Input: part model. Units: mm. Frame: model coordinates. Face numbers are marked on the shaded views. Round coordinates to 2 decimals unless told otherwise and drop trailing zeros. Order: outer loops, then holes, each group sorted by start corner. A loop starts at its lowest first (then second) coordinate and runs counter-clockwise, first axis right, second up. Notation, with made-up numbers: (-34.75, 56.5) -> (8.25, 56.5) arc R22 ccw to (8.25, 92.5) -> close; hole circle Ø2 at (-21.75, 58.25). An arc over 180 degrees is marked (long way). Use a Markdown table: item, result.
from build123d import *

# Parameters (mm, degrees)
SKETCH1_W                = 21.59
SKETCH1_H                = 13.97
DEPTH_A_DEPTH            = 6.35
ROUND_EXTRUDE_DEPTH      = 21.59
ANGLE_CUT_DEPTH          = 29.967416609
STRING_HOLE_R            = 0.762
STRING_HOLE_CUT_DEPTH    = 29.967416609
ELASTIC_HOLES_R          = 2.54
ELASTIC_HOLE_CUT_DEPTH   = 29.967416609
FILLET1_R                = 6.35
GUIDE_OUTIE_REACH        = 30.967
SKETCH7_R                = 2.54
ELASTIC_HOLE_CUT_2_DEPTH = 29.967416778


with BuildPart() as part:
    # Sketch1 → depth a (new body)
    with BuildSketch(Plane(origin=(0, 0, 0), x_dir=(1, 0, 0), z_dir=(0, 1, 0))):
        with Locations((-10.795, 6.985)):
            Rectangle(SKETCH1_W, SKETCH1_H)
    extrude(amount=DEPTH_A_DEPTH)

    # Sketch4 → round extrude (add)
    with BuildSketch(Plane(origin=(0, 0, 0), x_dir=(0, 0, -1), z_dir=(1, 0, 0))):
        with BuildLine():
            Line((0, 6.35), (13.97, 6.35))
            ThreePointArc((13.97, 6.35), (6.985, 13.335), (0, 6.35))
        make_face()
    extrude(amount=-ROUND_EXTRUDE_DEPTH)

    # Sketch5 → angle cut (cut, through all)
    with BuildSketch(Plane.XY):
        Polygon((0, 6.35), (0, 13.335), (-6.985, 13.335), align=None)
    extrude(amount=-ANGLE_CUT_DEPTH, mode=Mode.SUBTRACT)

    # string hole → string hole cut (cut, through all)
    with BuildSketch(Plane(origin=(0, 0, 0), x_dir=(0, 0, -1), z_dir=(1, 0, 0))):
        with Locations((6.985, 11.684)):
            Circle(STRING_HOLE_R)
    extrude(amount=-STRING_HOLE_CUT_DEPTH, mode=Mode.SUBTRACT)

    # elastic holes → elastic hole cut (cut, through all)
    with BuildSketch(Plane(origin=(0, 0, 0), x_dir=(0, 0, -1), z_dir=(1, 0, 0))):
        with Locations((3.4925, 3.175)):
            Circle(ELASTIC_HOLES_R)
        with Locations(Location((10.4775, 3.175, 0), (0, 0, 180))):
            Circle(ELASTIC_HOLES_R)
    extrude(amount=-ELASTIC_HOLE_CUT_DEPTH, mode=Mode.SUBTRACT)

    # Fillet1
    # the kernel refuses this fillet: 6.35 mm, written as the material it takes off along each edge
    with BuildSketch(Plane(origin=(-21.59, 6.35, -6.985), x_dir=(0, 0, -1), z_dir=(0, -1, 0))) as fillet1_piece_1:
        with BuildLine():
            CenterArc((6.985 - FILLET1_R, FILLET1_R), FILLET1_R, 270, 90)
            Line((6.985, FILLET1_R), (6.985, 0))
            Line((6.985, 0), (6.985 - FILLET1_R, 0))
        make_face()
    revolve(axis=Axis((-21.59, 6.35, -6.985), (1, 0, 0)), revolution_arc=180, mode=Mode.SUBTRACT)
    with BuildSketch(Plane(origin=(-21.59, -15.875, 0), x_dir=(1, 0, 0), z_dir=(0, 1, 0)), Plane(origin=(-21.59, -15.875, -13.97), x_dir=(0, 0, 1), z_dir=(0, 1, 0))) as fillet1_piece_2:
        with BuildLine():
            CenterArc((FILLET1_R, FILLET1_R), FILLET1_R, 180, 90)
            Line((0, FILLET1_R), (0, 0))
            Line((0, 0), (FILLET1_R, 0))
        make_face()
    extrude(amount=22.225, mode=Mode.SUBTRACT)

    # guide outie: up to this plane
    guide_outie_end = Plane(origin=(-6.985, 13.335, -13.97), z_dir=(-0.7071067811865512, -0.7071067811865439, 0))
    # guide → guide outie (add, up to the surface)
    with BuildSketch(Plane(origin=(0, 0, 0), x_dir=(1, 0, 0), z_dir=(0, 1, 0)), mode=Mode.PRIVATE) as guide_outie_sk1:
        with BuildLine():
            Line((0, 13.97), (0, 0))
            ThreePointArc((0, 0), (2.781966725, 6.985), (0, 13.97))
        make_face()
    guide_outie_tool1 = split(extrude(guide_outie_sk1.sketch, amount=GUIDE_OUTIE_REACH, mode=Mode.PRIVATE), bisect_by=guide_outie_end, keep=Keep.BOTH, mode=Mode.PRIVATE)
    add(guide_outie_tool1.solids().sort_by_distance((1.126975, 0, -6.985))[0])

    # Sketch7 → elastic hole cut 2 (cut, through all)
    with BuildSketch(Plane.ZY):
        with Locations(Location((-3.4925, 3.175, 0), (0, 0, 169.990167885))):
            Circle(SKETCH7_R)
        with Locations(Location((-10.4775, 3.175, 0), (0, 0, 180))):
            Circle(SKETCH7_R)
    extrude(amount=-ELASTIC_HOLE_CUT_2_DEPTH, mode=Mode.SUBTRACT)


solid = part.part
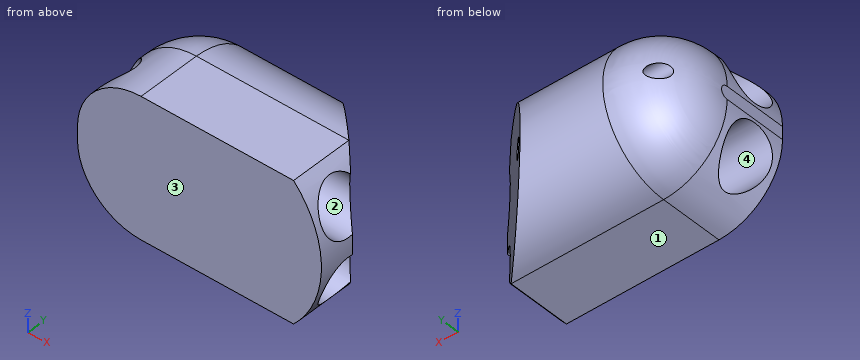
1) Ray query, probe 1 along Z at (x, y) = (-12.25, 1.5); probe 2 along Z at (x, y) = (-9, 4); probe 3 along Y at (x, z) = (-9, -7). Return the intervals inside material, ascending.
Answer key:
| item | result |
|---|---|
| probe 1 | z = -13.97 to -12.39, -8.57 to -5.4, -1.58 to 0 |
| probe 2 | z = -13.97 to -12.88, -8.08 to -5.89, -1.09 to 0 |
| probe 3 | y = 0 to 10.92, 12.45 to 13.33 |
2) Cut plane B-B on x = -14.25. State how many separate pieces and enclosed holes the cut face has, and give its area (3 significant figures).
Answer key:
| item | result |
|---|---|
| separate pieces | 1 |
| enclosed holes | 3 |
| area | 123 mm^2 |
3) Cut plane A-A on y = 4. Return loops of the section in (x, z) (3 decimals), and give its area (3 significant figures).
Answer key:
| item | result |
|---|---|
| outline | (-21.59, -7.62) arc R6.35 ccw to (-21.574, -8.075) -> (2.35, -8.075) -> (2.35, -5.895) -> (-21.574, -5.895) arc R6.35 ccw to (-21.59, -6.35) -> close; (-18.798, -12.88) arc R6.35 ccw to (-15.24, -13.97) -> (0, -13.97) arc R10.16 ccw to (0.897, -12.88) -> close; (-18.798, -1.09) -> (0.897, -1.09) arc R10.16 ccw to (0, 0) -> (-15.24, 0) arc R6.35 ccw to start |
| area | 91.7 mm^2 |
4) Contact query for flat-ended pins moving along their axis: P1, Ø1.5, axis at y = 11, z = -7, coming from the +X side; P2, Ø0.9, axis at y = 11.684, z = -6.985, coming from the -X side; P3, Ø5, axis at x = -8, z = -12.5, coming from the +Y side; P4, Ø6.5, axis at y = 3.18, z = -10.48, coming from the -X side. Output: stop coordinate, or through.
Answer key:
| item | result |
|---|---|
| P1 | stops at x = -3.9 |
| P2 | passes through |
| P3 | stops at y = 12.65 |
| P4 | stops at x = -21.59 |
5) Draft query along Y for the marked faces 1, 2, 3 and 4. Return one class per face: released by +Y, released by -Y, zero draft, split by the parting line, or undercut.
Answer key:
| item | result |
|---|---|
| face 1 | zero draft |
| face 2 | undercut |
| face 3 | released by -Y |
| face 4 | undercut |
